Model file for the job. Use its own axes, mm. Face numbers are marked on the shaded views. A direction names the side the tool comes from. Coordinates: 2 decimals unless noted, no trailing zeros. Write each loop counter-clockwise with the first axis right and the second up, starting at its lowest first coordinate (ties: lowest second). Pieces come first, ordered by that corner, then holes. Notation, with made-up numbers: (21, 73) -> (52, 73) arc R27 cw to (52, 102) -> close; hole circle Ø10 at (-14.5, 83). An arc over 180 degrees is marked (long way). Answer as a JSON object with one key per item and string values. Group by question number.
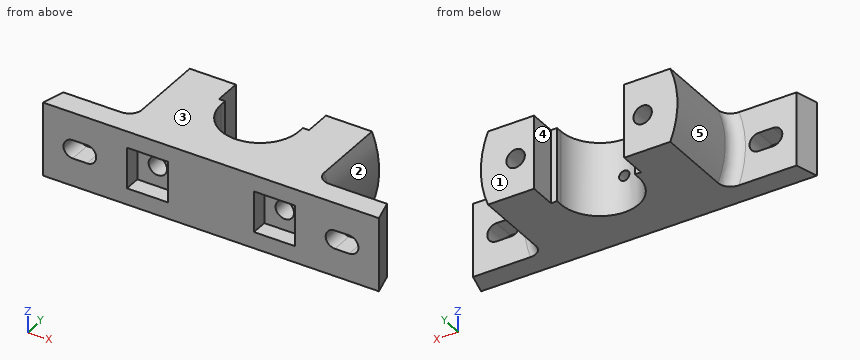
from build123d import *

# Parameters (mm, degrees)
BOSS_EXTRUDE3_DEPTH   = 18
CUT_EXTRUDE1_DEPTH    = 43
M6_TAPPED_HOLE1_D     = 5
M6_TAPPED_HOLE1_DEPTH = 6
M6_TAPPED_HOLE1_TIP   = 1.502151548
M10_TAPPED_HOLE1_D    = 9
SKETCH9_W             = 20
SKETCH9_H             = 20
CUT_EXTRUDE2_DEPTH    = 8
CUT_EXTRUDE3_DEPTH    = 11
FILLET2_R             = 6
FILLET3_R             = 6


with BuildPart() as part:
    # Sketch1 → Boss-Extrude3 (new body, symmetric)
    with BuildSketch(Plane.XY):
        with BuildLine():
            Line((-82, -43.82348407), (82, -43.82348407))
            Line((82, -43.82348407), (79, -32.82348407))
            Line((79, -32.82348407), (50, -32.82348407))
            Line((50, -32.82348407), (50, 10.17651593))
            Line((50, 10.17651593), (22, 10.17651593))
            Line((22, 10.17651593), (22, -2.82348407))
            Line((22, -2.82348407), (19, -2.82348407))
            Line((19, -2.82348407), (19, -5.82348407))
            ThreePointArc((19, -5.82348407), (0, -24.82348407), (-19, -5.82348407))
            Line((-19, -5.82348407), (-19, -2.82348407))
            Line((-19, -2.82348407), (-22, -2.82348407))
            Line((-22, -2.82348407), (-22, 10.17651593))
            Line((-22, 10.17651593), (-50, 10.17651593))
            Line((-50, 10.17651593), (-50, -32.82348407))
            Line((-50, -32.82348407), (-79, -32.82348407))
            Line((-79, -32.82348407), (-82, -43.82348407))
        make_face()
    extrude(amount=BOSS_EXTRUDE3_DEPTH, both=True)

    # Sketch3 → Cut-Extrude1 (cut)
    with BuildSketch(Plane(origin=(0, 10.17651593, 0), x_dir=(1, 0, 0), z_dir=(0, 1, 0))):
        with BuildLine():
            Line((-44.497190923, 18), (-50, 18))
            Line((-50, 18), (-50, -18))
            Line((-50, -18), (-44.497190923, -18))
            ThreePointArc((-44.497190923, -18), (-48, 0), (-44.497190923, 18))
        make_face()
    cut_extrude1 = extrude(amount=-CUT_EXTRUDE1_DEPTH, mode=Mode.SUBTRACT)

    # Mirror1: Cut-Extrude1 across plane
    add(cut_extrude1.mirror(Plane(origin=(0, 0, 0), x_dir=(0, 0, 1), z_dir=(1, 0, 0))), mode=Mode.SUBTRACT)

    # M6 Tapped Hole1
    with Locations(Plane(origin=(0, -24.82348407, 0), x_dir=(1, 0, 0), z_dir=(0, 1, 0))):
        with Locations((0, 0)):
            Hole(M6_TAPPED_HOLE1_D / 2, depth=M6_TAPPED_HOLE1_DEPTH)
            with Locations((0, 0, -(M6_TAPPED_HOLE1_DEPTH + M6_TAPPED_HOLE1_TIP / 2))):  # 118° drill point
                Cone(0, M6_TAPPED_HOLE1_D / 2, M6_TAPPED_HOLE1_TIP, mode=Mode.SUBTRACT)

    # M10 Tapped Hole1 (through all)
    with Locations(Plane(origin=(0, 10.17651593, 0), x_dir=(1, 0, 0), z_dir=(0, 1, 0))):
        with Locations((-31, 0)):
            m10_tapped_hole1 = Hole(M10_TAPPED_HOLE1_D / 2)

    # Sketch9 → Cut-Extrude2 (cut)
    with BuildSketch(Plane.XZ.offset(43.82348407)):
        with Locations((-31, 0)):
            Rectangle(SKETCH9_W, SKETCH9_H)
    cut_extrude2 = extrude(amount=-CUT_EXTRUDE2_DEPTH, mode=Mode.SUBTRACT)

    # Sketch10 → Cut-Extrude3 (cut)
    with BuildSketch(Plane.XZ.offset(43.82348407)):
        with BuildLine():
            Line((-67.5, 4.5), (-60.5, 4.5))
            ThreePointArc((-60.5, 4.5), (-56, 0), (-60.5, -4.5))
            Line((-60.5, -4.5), (-67.5, -4.5))
            ThreePointArc((-67.5, -4.5), (-72, 0), (-67.5, 4.5))
        make_face()
    cut_extrude3 = extrude(amount=-CUT_EXTRUDE3_DEPTH, mode=Mode.SUBTRACT)

    # Mirror2: M10 Tapped Hole1, Cut-Extrude2, Cut-Extrude3 across plane
    add(m10_tapped_hole1.mirror(Plane(origin=(0, 0, 0), x_dir=(0, 0, 1), z_dir=(1, 0, 0))), mode=Mode.SUBTRACT)
    add(cut_extrude2.mirror(Plane(origin=(0, 0, 0), x_dir=(0, 0, 1), z_dir=(1, 0, 0))), mode=Mode.SUBTRACT)
    add(cut_extrude3.mirror(Plane(origin=(0, 0, 0), x_dir=(0, 0, 1), z_dir=(1, 0, 0))), mode=Mode.SUBTRACT)

    # Fillet2
    fillet2_edges = [part.edges().sort_by_distance(p)[0] for p in [
        (-48, -32.82348407, 0),
    ]]
    fillet(fillet2_edges, radius=FILLET2_R)

    # Fillet3
    fillet3_edges = [part.edges().sort_by_distance(p)[0] for p in [
        (48, -32.82348407, 0),
    ]]
    fillet(fillet3_edges, radius=FILLET3_R)


solid = part.part
(1) Cut at C-C on x = 65. List the corners of the cut face in (y, z), plus the area to 3 significant figures.
(2) 3-axis set-ups, long thin cutter, end or side, ignore diameter. For the marked faces 1 and 2: which of +Z, -Z, +X, -X, +Y, -Y reach the whole face in a straight line?
(3) Pull direction Z, two halves, no side cores. Call the marked faces 3, 4 and 5: released by +Z, released by -Z, zero draft, split by the parting line, or undercut.
(4) Cut at D-D on x = 33. List the corners of the cut face in (y, z).
(5) Wall check: probe 1 along Z at (x, y) = (31, -3); probe 2 along X at (y, z) = (-8, 3); probe 3 along X at (y, z) = (-3.5, -3). Give the ranges that are in metal, low to high.
(6) Cut at A-A on x = -31. List the corners of the cut face in (y, z).
(7) Cut at B-B on y = -13. List the corners of the cut face in (x, z).
(8) Pin check, flat tips, straight feed: pin 1 (2.5 mm diameter, centred on y = -39, z = 2.5, fed in from +X); pin 2 (10.5 mm diameter, centred on y = 4.5, z = -7, fed in from +X); pin 3 (8 mm diameter, centred on y = -10.5, z = -9, fed in from -X). Stop position of each tip, or through.
Results found:
{
 "1": {"outline": "(-43.82, -18) -> (-32.82, -18) -> (-32.82, -4.5) -> (-43.82, -4.5) -> close; (-43.82, 4.5) -> (-32.82, 4.5) -> (-32.82, 18) -> (-43.82, 18) -> close", "area": "297 mm²"},
 "2": {"face 1": "+Z, -Z, +X, -X, +Y", "face 2": "+X, +Y"},
 "3": {"face 3": "released by +Z", "face 4": "zero draft", "face 5": "split by the parting line"},
 "4": {"outline": "(-43.82, -18) -> (10.18, -18) -> (10.18, -4.03) -> (-35.82, -4.03) -> (-35.82, -10) -> (-43.82, -10) -> close; (-43.82, 10) -> (-35.82, 10) -> (-35.82, 4.03) -> (10.18, 4.03) -> (10.18, 18) -> (-43.82, 18) -> close"},
 "5": {"probe 1": "z = -18 to -4.5, 4.5 to 18", "probe 2": "x = -47.91 to -34.35, -27.65 to -18.87, 18.87 to 27.65, 34.35 to 47.91", "probe 3": "x = -47.91 to -34.35, -27.65 to -19, 19 to 27.65, 34.35 to 47.91"},
 "6": {"outline": "(-43.82, -18) -> (10.18, -18) -> (10.18, -4.5) -> (-35.82, -4.5) -> (-35.82, -10) -> (-43.82, -10) -> close; (-43.82, 10) -> (-35.82, 10) -> (-35.82, 4.5) -> (10.18, 4.5) -> (10.18, 18) -> (-43.82, 18) -> close"},
 "7": {"outline": "(-44.5, -18) -> (-17.59, -18) -> (-17.59, 18) -> (-44.5, 18) arc R48 ccw to start; (17.59, -18) -> (44.5, -18) arc R48 ccw to (44.5, 18) -> (17.59, 18) -> close; hole circle Ø9 at (-31, 0); hole circle Ø9 at (31, 0)"},
 "8": {"pin 1": "stops at x = 81.03", "pin 2": "stops at x = 47.97", "pin 3": "stops at x = -47.74"}
}
